Could you check a few things on this model? Use its own coordinates, in mm. A direction names the side the tool comes from. Round coordinates to 2 decimals unless told otherwise and drop trailing zeros. Write each loop counter-clockwise with the first axis right and the second up, starting at its lowest first coordinate (ties: lowest second). Pieces come first, ordered by that corner, then holes. Notation, with made-up numbers: (70.25, 10) -> (112.25, 10) arc R22 ccw to (112.25, 16) -> close; hole circle Ø10 at (-2, 65). An arc over 180 degrees is marked (long way). One line per question, with ' | ' between items. Start each with the question number.
1. For faces 1 (the flat face through (-6, 2, 8)), 2 (the flat face through (-1, 5, 16.7)), 3 (the flat face through (-4, 2, 16.7)), which set-ups out of +Z, -Z, +X, -X, +Y, -Y let a thin tool reach every point of the face, with its end or its side?
2. Imagine slicing it at C-C, the plane y = 18.25. List the corners of the cut face in (x, z) for me.
3. Imagine slicing it at B-B, the plane y = 11. List the corners of the cut face in (x, z) for me, and give its area (3 significant figures).
4. Imagine slicing it at D-D, the plane z = 17.7. List the corners of the cut face in (x, y) for me, and give its area (3 significant figures).
5. Imagine slicing it at A-A, the plane z = 6. List the corners of the cut face in (x, y) for me.
6. If I drill on line 1 along Y through (x, z) = (-1.15, 17.7); line 2 along Y through (x, z) = (-3, 15.5); line 3 along X through (y, z) = (5.25, 20), over which ranges is the centre line in solid material (lowest first)? Write a range as [from, to].
7. For pin 1 Ø1.5 at (y, z) = (2, 11.5) entering from -X; pin 2 Ø6 at (x, y) = (-6.5, 9) entering from -Z; pin 3 Ø3 at (x, y) = (-3, 14.5) entering from +Z; pin 4 Ø1 at (x, y) = (1.5, 8.5) entering from -Z, each with a flat end and sliding along its axis, tell me the tip position at first contact or that it passes through.
8. Thinking about a two-plate mould opening in Z: for faces 4 (the flat face through (-2.741, 8.402, 24.236)), 5 (the flat face through (-1, 17, 16.7)), 6 (the flat face through (-6, 21, 8)), which applies, released by +Z, released by -Z, zero draft, split by the parting line, or undercut?
Autodesk Inventor part; units mm, degrees
ref_plane "YZ Plane" through (0, 0, 0) normal (1, 0, 0) x (0, 1, 0)
ref_plane "XZ Plane" through (0, 0, 0) normal (0, 1, 0) x (-1, 0, 0)
ref_plane "XY Plane" through (0, 0, 0) normal (0, 0, 1) x (1, 0, 0)
sketch "Sketch1" plane through (0, 0, 0) normal (0, 1, 0) x (-1, 0, 0)
  line L0 (0, 0) -> (2, 0)
  line L1 (2, 0) -> (2, 22.2)
  line L2 (2, 22.2) -> (0, 22.2)
  line L3 (0, 22.2) -> (0, 0)
  line L4 (0.1206, 22.884) -> (2, 22.2)
  line L5 (2, 22.2) -> (4.7362, 29.7175)
  line L6 (4.7362, 29.7175) -> (2.8568, 30.4016)
  line L7 (2.8568, 30.4016) -> (0.1206, 22.884)
  line L8 (2, 22.2) -> (-13.9637, 28.0103) construction
  line L9 (3.7965, 30.0596) -> (1.0603, 22.542) construction
  arc A0 (2.684, 24.0794) -> (2, 20.2) centre (2, 22.2) ccw
  arc A1 (2, 20.2) -> (2.684, 24.0794) centre (2, 22.2) ccw
  circle A2 centre (3.7965, 30.0596) radius 3.9783
  circle A3 centre (1, 0) radius 3.8044
  dimension "d0" = 2
  dimension "d1" = 22.2
  dimension "d26" = 2
  dimension "d27" = 20
  dimension "d28" = 8
extrude "Extrusion6" add sketch "Sketch1" along normal blind 22 contours L3 A3 L1 L0 | L3 A0 L1 A3 | A0 L4 L2 | L2 L1 A0 | L1 L5 A1 | L4 A0 L5 | L7 A2 L5 A0 | L7 L6 L5 A2 picked at (1.1123, 1.2632) picked at (3.2392, 28.8563)
extrude "Extrusion7" cut sketch "Sketch1" along normal blind 22 contours L1 L5 A1
sketch "Sketch4" plane through (-4.7362, 0, 29.7175) normal (-0.9397, 0, -0.342) x (-0.342, 0, 0.9397)
  line L0 (-8, 22) -> (0, 22)
  line L1 (-8, 0) -> (-8, 22)
  circle A0 centre (-4, 11) radius 2.7
  point P0 (-29.5452, 0)
  point P1 (-8, 11)
  point P2 (-4, 22)
  dimension "d33" = 5.4
extrude "Extrusion8" cut sketch "Sketch4" against normal blind 3
sketch "Sketch5" plane through (-2, 0, 0) normal (-1, 0, 0) x (0, 0, 1)
  line L0 (0, 22) -> (22.2, 22)
  line L1 (0, 0) -> (0, 22)
  line L2 (0, 0) -> (22.2, 0)
  line L3 (22.2, 0) -> (22.2, 22)
  circle A0 centre (17.7, 11) radius 4.7
  line L4 (16.7, 22) -> (16.7, 0) construction
  line L5 (0, 19) -> (16.7, 19)
  line L6 (16.7, 19) -> (16.7, 3)
  line L7 (16.7, 3) -> (0, 3)
  line L8 (0, 3) -> (0, 19)
  line L9 (0, 22) -> (16.7, 22)
  line L10 (16.7, 22) -> (16.7, 19)
  line L11 (16.7, 19) -> (0, 19)
  line L12 (0, 19) -> (0, 22)
  line L13 (0, 3) -> (16.7, 3)
  line L14 (16.7, 3) -> (16.7, 0)
  line L15 (16.7, 0) -> (0, 0)
  line L16 (0, 0) -> (0, 3)
  point P0 (22.2, 11)
  point P1 (16.7, 11)
  point P2 (0, 11)
  dimension "d36" = 9.4
  dimension "d37" = 4.5
  dimension "d38" = 16.7
  dimension "d39" = 16
extrude "Extrusion9" cut sketch "Sketch5" against normal blind 3 contours L5 L6 A0 L7 L1 | A0 L3 | L3 A0 L6 | L6 A0
extrude "Extrusion11" add sketch "Sketch1" along normal blind 0.6 contours L3 A3 L1 L0 | L0 L1 A3 L3 | A2 L5 L6 L7 | L7 L6 L5 A2
extrude "Extrusion12" add sketch "Sketch5" along normal blind 4 contours L0 L10 L5 L1 | L7 L14 L2 L1
equation "\"sp\" = 0.4"
properties part number "EncoderBracket"
Geometry results:
1) face 1: -Z, -X, +Y, -Y | face 2: -Z, +X, -X | face 3: -X, +Y, -Y
2) outline: (-4.74, 29.72) -> (-2, 22.2) -> (-2, 16.7) -> (0, 16.7) -> (0, 22.2) arc R2 ccw to (-0.12, 22.88) -> (-2.86, 30.4) -> close
3) outline: (-4.74, 29.72) -> (-4.29, 28.5) -> (-2.41, 29.18) -> (-2.86, 30.4) -> close; (-2.44, 23.42) -> (-2, 22.2) -> (-2, 22.4) -> (-0.01, 22.4) arc R2 ccw to (-0.12, 22.88) -> (-0.57, 24.11) -> close | area: 5.50 mm2
4) outline: (-2, 0) -> (0, 0) -> (0, 6.3) -> (-2, 6.3) -> close; (-2, 15.7) -> (0, 15.7) -> (0, 22) -> (-2, 22) -> close | area: 25.2 mm2
5) outline: (-6, 0) -> (0, 0) -> (0, 3) -> (-6, 3) -> close; (-6, 19) -> (0, 19) -> (0, 22) -> (-6, 22) -> close
6) line 1: y = [0, 6.3], [15.7, 22] | line 2: y = [0, 3], [19, 22] | line 3: x = [-2, 0]
7) pin 1: stops at x = -6 | pin 2: stops at z = 26.51 | pin 3: stops at z = 30.4 | pin 4: passes through
8) face 4: undercut | face 5: released by -Z | face 6: zero draft
